Design review of the part built by this model. Coordinates are the model's own, in mm. Face numbers are marked on the shaded views. A direction names the side the tool comes from. Give positions to 0.01 mm unless a question says otherwise; leave off trailing zeros. Write each loop counter-clockwise with the first axis right and the second up, starting at its lowest first coordinate (ties: lowest second). Pieces come first, ordered by that corner, then holes. Notation, with made-up numbers: (83.5, 6) -> (120.5, 6) arc R9 cw to (120.5, 19) -> close; hole circle Ø4 at (45.5, 6.25). An arc over 180 degrees is marked (long way). Return JSON: item names as keys, results as strings. Group by question number.
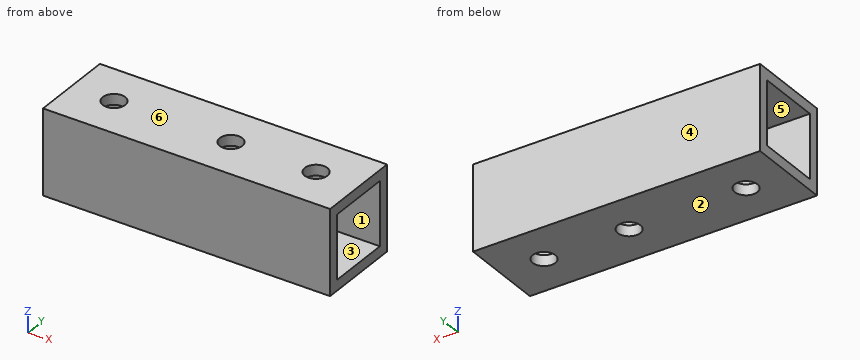
Autodesk Inventor part; units mm, degrees
ref_plane "YZ Plane" through (0, 0, 0) normal (1, 0, 0) x (0, 1, 0)
ref_plane "XZ Plane" through (0, 0, 0) normal (0, 1, 0) x (-1, 0, 0)
ref_plane "XY Plane" through (0, 0, 0) normal (0, 0, 1) x (1, 0, 0)
sketch "Sketch1" plane through (0, 0, 0) normal (1, 0, 0) x (0, 1, 0)
  line L0 (0, 0) -> (25.4, 0)
  line L1 (25.4, 0) -> (25.4, 25.4)
  line L2 (25.4, 25.4) -> (0, 25.4)
  line L3 (0, 25.4) -> (0, 0)
  line L4 (3.175, 22.225) -> (22.225, 22.225)
  line L5 (22.225, 22.225) -> (22.225, 3.175)
  line L6 (22.225, 3.175) -> (3.175, 3.175)
  line L7 (3.175, 3.175) -> (3.175, 22.225)
  dimension "d0" = 25.4
  dimension "d1" = 25.4
  dimension "d2" = 3.175
extrude "Extrusion1" add sketch "Sketch1" along normal blind 85.725
sketch "Sketch2" plane through (0, 0, 25.4) normal (0, 0, 1) x (1, 0, 0)
  circle A0 centre (12.7, 12.7) radius 3.3734
  circle A1 centre (73.025, 12.7) radius 3.3734
  line L0 (85.725, 25.4) -> (85.725, 0)
  line L1 (0, 0) -> (85.725, 0)
  line L2 (0, 25.4) -> (0, 0)
  circle A2 centre (47.625, 12.7) radius 3.3734
  line L3 (0, 25.4) -> (85.725, 25.4)
  dimension "d5" = 6.7469
  dimension "d6" = 6.7469
  dimension "d7" = 12.7
  dimension "d8" = 12.7
  dimension "d9" = 12.7
  dimension "d10" = 12.7
  dimension "d13" = 6.7469
  dimension "d15" = 12.7
  dimension "d16" = 25.4
extrude "Extrusion2" cut sketch "Sketch2" against normal blind 25.4 contours A0 | A1 | A2
properties part number "support block 2"
Q1. Mouldability with a two-part tool opening along Y and no side actions: class the marked faces 1, 2, 3 and 4 as +Y half, -Y half, draft (parallel to the pull), parting line (faces both ways), or undercut.
Q2. Take a section at D-D, the plane x = 12.7. Give the boundary of the cut face in (y, z) (3 decimals).
Q3. Take a section at B-B, the plane z = 6. Give the boundary of the cut face in (x, y) (3 decimals).
Q4. Tool access review of the marked faces 5 and 6: name each direction out of +Z, -Z, +X, -X, +Y, -Y from which nothing blocks a thin tool from reaching the whole face with its end or side.
Q5. Take a section at A-A, the plane y = 12.7. Count the separate pieces of the cut face and the enclosed holes in it, plus the area to 3 significant figures.
Q6. For L1, parallel to Z at x = 16, y = 3.25 (3 decimals), list the stretches that pass through material, from the lowest coordinate up. Write a range as from..to.
Q7. Insertion check: pin 1 (3 mm diameter, centred on y = 19.5, z = 11, fed in from +X). The pin has a flat end and moves straight along its axis. Give the tip position at first contact, or say it passes through.
Final values:
{
 "1": {"face 1": "undercut", "face 2": "draft", "face 3": "undercut", "face 4": "+Y half"},
 "2": {"outline": "(0, 0) -> (9.327, 0) -> (9.327, 3.175) -> (3.175, 3.175) -> (3.175, 22.225) -> (9.327, 22.225) -> (9.327, 25.4) -> (0, 25.4) -> close; (16.073, 0) -> (25.4, 0) -> (25.4, 25.4) -> (16.073, 25.4) -> (16.073, 22.225) -> (22.225, 22.225) -> (22.225, 3.175) -> (16.073, 3.175) -> close"},
 "3": {"outline": "(0, 0) -> (85.725, 0) -> (85.725, 3.175) -> (0, 3.175) -> close; (0, 22.225) -> (85.725, 22.225) -> (85.725, 25.4) -> (0, 25.4) -> close"},
 "4": {"face 5": "+X, -X", "face 6": "+Z, +X, -X, +Y, -Y"},
 "5": {"separate pieces": "8", "enclosed holes": "0", "area": "416 mm²"},
 "6": {"L1": "z = 0..3.175, 22.225..25.4"},
 "7": {"pin 1": "passes through"}
}
